The listing builds one solid part. Answer for the finished solid, in the listing's coordinates (mm). A direction names the side the tool comes from. Give positions to 0.01 mm unless a question says otherwise; leave off trailing zeros. Order: outer loops, then holes, each group sorted by start corner. A loop starts at its lowest first (then second) coordinate and runs counter-clockwise, first axis right, second up. Notation, with made-up numbers: M 27.5,-29 L 42.5,-29 A17 ccw 42.5,-6 Z; hole C 81.25,58 d10. An arc over 180 degrees is marked long. Answer as a JSON object with one key per item and string values. Group by question number.
```python
from build123d import *

# Parameters (mm, degrees)
SKETCH_1_R               = 19.5
SKETCH_1_R_2             = 18
EXTRUDE_1_DEPTH          = 20
SKETCH_3_R               = 27.5
EXTRUDE_2_DEPTH          = 3
SKETCH_10_R              = 6
SKETCH_10_R_2            = 5
EXTRUDE_6_DEPTH          = 10
SKETCH_11_R              = 5.007506695
CUT_EXTRUDE_4_DEPTH      = 19
CUT_EXTRUDE_4_DEPTH_BACK = 10
SKETCH_15_W              = 20
SKETCH_15_H              = 60
SKETCH_15_W_2            = 13
SKETCH_15_H_2            = 25
EXTRUDE_7_DEPTH          = 1
EXTRUDE_7_DEPTH_BACK     = 2
SKETCH_16_W              = 5
SKETCH_16_H              = 5
EXTRUDE_8_DEPTH          = 10
SKETCH_18_R              = 0.875
CUT_EXTRUDE_5_DEPTH      = 10
CUT_EXTRUDE_5_DEPTH_BACK = 39
SKETCH_12_W              = 21.5
SKETCH_12_H              = 13
CUT_EXTRUDE_6_DEPTH      = 21.5
SKETCH_19_W              = 22.5
SKETCH_19_H              = 14
SKETCH_19_W_2            = 21.5
SKETCH_19_H_2            = 13
EXTRUDE_9_DEPTH          = 10
FILLET_2_R               = 1
FILLET_3_R               = 1
FILLET_4_R               = 1
FILLET_5_R               = 1
SKETCH_25_R              = 21.75
SKETCH_25_R_2            = 19.5
EXTRUDE_12_DEPTH         = 2
EXTRUDE_START            = -1
SKETCH_26_R              = 21.75
SKETCH_26_R_2            = 19.5
EXTRUDE_13_DEPTH         = 2


with BuildPart() as part:
    # 草圖1 → 填料-伸長1 (new body)
    with BuildSketch(Plane(origin=(0, 0, 0), x_dir=(1, 0, 0), z_dir=(0, 1, 0))):
        Circle(SKETCH_1_R)
        Circle(SKETCH_1_R_2, mode=Mode.SUBTRACT)
    extrude(amount=EXTRUDE_1_DEPTH)

    # 草圖3 → 填料-伸長2 (add)
    with BuildSketch(Plane.XZ):
        Circle(SKETCH_3_R)
    extrude(amount=EXTRUDE_2_DEPTH)

    # 草圖10 → 填料-伸長6 (add)
    with BuildSketch(Plane(origin=(0, -3, 0), x_dir=(-1, 0, 0), z_dir=(0, -1, 0))):
        with Locations((0, 11.196036894)):
            Circle(SKETCH_10_R)
        with Locations((0, 11.196036894)):
            Circle(SKETCH_10_R_2, mode=Mode.SUBTRACT)
    extrude(amount=-EXTRUDE_6_DEPTH)

    # 草圖11 → 除料-伸長4 (cut, two sides)
    with BuildSketch(Plane(origin=(0, -3, 0), x_dir=(-1, 0, 0), z_dir=(0, -1, 0))) as cut_extrude_4_sk:
        with Locations((0, 11.196036894)):
            Circle(SKETCH_11_R)
    extrude(amount=CUT_EXTRUDE_4_DEPTH, mode=Mode.SUBTRACT)
    extrude(cut_extrude_4_sk.sketch, amount=-CUT_EXTRUDE_4_DEPTH_BACK, mode=Mode.SUBTRACT)

    # 草圖15 → 填料-伸長7 (add, two sides)
    with BuildSketch(Plane.XY.offset(-3)) as extrude_7_sk:
        with Locations((0, -33)):
            Rectangle(SKETCH_15_W, SKETCH_15_H)
        with Locations((0, -40.5)):
            Rectangle(SKETCH_15_W_2, SKETCH_15_H_2, mode=Mode.SUBTRACT)
    extrude(amount=EXTRUDE_7_DEPTH)
    extrude(extrude_7_sk.sketch, amount=-EXTRUDE_7_DEPTH_BACK)

    # 草圖16 → 填料-伸長8 (add)
    with BuildSketch(Plane.XY.offset(-3)):
        with Locations((0, -25.5)):
            Rectangle(SKETCH_16_W, SKETCH_16_H)
        with Locations((0, -55.5)):
            Rectangle(SKETCH_16_W, SKETCH_16_H)
    extrude(amount=-EXTRUDE_8_DEPTH)

    # 草圖18 → 除料-伸長5 (cut, two sides)
    with BuildSketch(Plane.XY) as cut_extrude_5_sk:
        with Locations((0, -55.5)):
            Circle(SKETCH_18_R)
        with Locations((0, -25.5)):
            Circle(SKETCH_18_R)
    extrude(amount=CUT_EXTRUDE_5_DEPTH, mode=Mode.SUBTRACT)
    extrude(cut_extrude_5_sk.sketch, amount=-CUT_EXTRUDE_5_DEPTH_BACK, mode=Mode.SUBTRACT)

    # 草圖12 → 除料-伸長6 (cut)
    with BuildSketch(Plane.XZ.offset(3)):
        with Locations((0, 6.907998134)):
            Rectangle(SKETCH_12_W, SKETCH_12_H)
    extrude(amount=-CUT_EXTRUDE_6_DEPTH, mode=Mode.SUBTRACT)

    # 草圖19 → 填料-伸長9 (add)
    with BuildSketch(Plane(origin=(0, 0, 0), x_dir=(1, 0, 0), z_dir=(0, 1, 0))):
        with Locations((0, -6.907998134)):
            Rectangle(SKETCH_19_W, SKETCH_19_H)
        with Locations((0, -6.907998134)):
            Rectangle(SKETCH_19_W_2, SKETCH_19_H_2, mode=Mode.SUBTRACT)
    extrude(amount=EXTRUDE_9_DEPTH)

    # 圓角2
    fillet_2_edges = [part.edges().sort_by_distance(p)[0] for p in [
        (-11.25, 5, -0.092001866),
    ]]
    fillet(fillet_2_edges, radius=FILLET_2_R)

    # 圓角3
    fillet_3_edges = [part.edges().sort_by_distance(p)[0] for p in [
        (11.25, 5, -0.092001866),
    ]]
    fillet(fillet_3_edges, radius=FILLET_3_R)

    # 圓角4
    fillet_4_edges = [part.edges().sort_by_distance(p)[0] for p in [
        (11.25, 5, 13.907998134),
    ]]
    fillet(fillet_4_edges, radius=FILLET_4_R)

    # 圓角5
    fillet_5_edges = [part.edges().sort_by_distance(p)[0] for p in [
        (-11.25, 5, 13.907998134),
    ]]
    fillet(fillet_5_edges, radius=FILLET_5_R)

    # 草圖25 → 填料-伸長12 (add)
    with BuildSketch(Plane(origin=(0, 7, 0), x_dir=(-1, 0, 0), z_dir=(0, -1, 0))):
        Circle(SKETCH_25_R)
        Circle(SKETCH_25_R_2, mode=Mode.SUBTRACT)
    extrude(amount=EXTRUDE_12_DEPTH)

    # 草圖26 → 填料-伸長13 (add)
    with BuildSketch(Plane(origin=(0, 10.5, 0), x_dir=(-1, 0, 0), z_dir=(0, -1, 0)).offset(EXTRUDE_START)):
        Circle(SKETCH_26_R)
        Circle(SKETCH_26_R_2, mode=Mode.SUBTRACT)
    extrude(amount=-EXTRUDE_13_DEPTH)


solid = part.part
```
Item 1: Section B-B (y = -35.5) is taken. Determine the outline of the cut face in (x, z).
Item 2: Section A-A (y = 8.5) is taken. Determine the outline of the cut face in (x, z), and give its area (3 significant figures).
Item 3: Section C-C (x = 14) is taken. Determine the outline of the cut face in (y, z), and give its area (3 significant figures).
Item 4: Consider probe 1 along Y at (x, z) = (0, -7.25) (3 decimals); probe 2 along Y at (x, z) = (15, 18.5); probe 3 along X at (y, z) = (10.25, 0). Determine where each line is inside the solid, lowest interval first. Write a range as from..to.
Item 5: A tool of negligible diameter and unlimited length cuts with its end or side. For faces 4 (the cylindrical face through (-2.539, 9.218, -19.334)), 5 (the flat face through (10.75, 3, 7)), 6 (the flat face through (1, 7, -6)), 7 (the flat face through (-6.5, -41, -3)), from which of +Z, -Z, +X, -X, +Y, -Y can it reach the whole face along a straight path? Write none if from no direction.
Item 6: Flat-ended cylindrical pins translate along their axes: P1, Ø6.5, axis at x = -1, y = 2, coming from the +Z side; P2, Ø1.5, axis at y = 4.5, z = -18.5, coming from the +X side; P3, Ø12, axis at x = -2, z = -6.5, coming from the -Y side; P4, Ø8, axis at y = 5, z = 9.5, coming from the -X side. Find the tip coordinate at first contact, or state that the pin passes through.
Item 7: Determine the mould class of faces 1 (the flat face through (2.5, -56, -9)), 2 (the flat face through (0, 0, -4)), 3 (the flat face through (8, 11.5, -18)) for opening direction X: released by +X, released by -X, zero draft, split by the parting line, or undercut.
Values found:
{
 "1": {"outline": "M -10,-5 L -6.5,-5 L -6.5,-2 L -10,-2 Z; M 6.5,-5 L 10,-5 L 10,-2 L 6.5,-2 Z"},
 "2": {"outline": "C 0,0 d39; M -11.25,0.91 A1 ccw -10.25,-0.09 L 10.25,-0.09 A1 ccw 11.25,0.91 L 11.25,12.91 A1 ccw 10.25,13.91 L -10.25,13.91 A1 ccw -11.25,12.91 Z; hole C 0,0 d36; hole M -10.75,0.41 L 10.75,0.41 L 10.75,13.41 L -10.75,13.41 Z", "area": "211 mm^2"},
 "3": {"outline": "M -3,-23.67 L 0,-23.67 L 0,-13.57 L 5,-13.57 L 5,-16.65 L 7,-16.65 L 7,-13.57 L 11.5,-13.57 L 11.5,-16.65 L 13.5,-16.65 L 13.5,-13.57 L 20,-13.57 L 20,-11.31 L 0,-11.31 L 0,11.31 L 20,11.31 L 20,13.57 L 13.5,13.57 L 13.5,16.65 L 11.5,16.65 L 11.5,13.57 L 7,13.57 L 7,16.65 L 5,16.65 L 5,13.57 L 0,13.57 L 0,23.67 L -3,23.67 Z", "area": "257 mm^2"},
 "4": {"probe 1": "y = -58..-56.375, -54.625..-53, -28..-26.375, -24.625..-23", "probe 2": "y = -3..0", "probe 3": "x = -19.5..-18, 18..19.5"},
 "5": {"face 4": "none", "face 5": "+Y, -Y", "face 6": "+Y", "face 7": "+Z, -Z"},
 "6": {"P1": "stops at z = 27.5", "P2": "stops at x = 12.3", "P3": "stops at y = -63", "P4": "stops at x = -21.04"},
 "7": {"face 1": "released by +X", "face 2": "undercut", "face 3": "zero draft"}
}
